```python
from build123d import *

# Parameters (mm, degrees)
F1_DEPTH = 6
F2_R     = 8
F2_R_2   = 7
F3_DEPTH = 5
F4_DEPTH = 26.3


with BuildPart() as f1:
    # F0 (on Front) → F1 (new body)
    with BuildSketch(Plane.XZ):
        Polygon((40, 0), (0, 0), (-40, 0), (-40, -29.434), (0, -29.434), (40, -29.434), align=None)
    extrude(amount=F1_DEPTH)

    # F2 (on face) → F3 (cut)
    with BuildSketch(Plane.XZ):
        with Locations((0, -8.284)):
            Circle(F2_R)
        with Locations((0, -8.284)):
            Circle(F2_R_2, mode=Mode.SUBTRACT)
    extrude(amount=F3_DEPTH, mode=Mode.SUBTRACT)

    # F2 (on face) → F4 (cut)
    with BuildSketch(Plane.XZ):
        with Locations((0, -8.284)):
            Circle(F2_R_2)
    extrude(amount=F4_DEPTH, mode=Mode.SUBTRACT)


solid = f1.part
```
Part model, mm, in its own coordinate system. A direction names the side the tool comes from. Coordinates: 2 decimals unless noted, no trailing zeros. Order: outer loops, then holes, each group sorted by start corner. A loop starts at its lowest first (then second) coordinate and runs counter-clockwise, first axis right, second up. Notation, with made-up numbers: (-25, 67.25) -> (8, 67.25) arc R26 cw to (8, 85.25) -> close; hole circle Ø2 at (68.25, 86.5). An arc over 180 degrees is marked (long way). Put each result on its own line as item: value. Start each with the question number.
(1) Probe line 1 along Z through (x, y) = (0, -2.15); line 2 along Z through (x, y) = (0, -5.4); line 3 along X through (y, z) = (-2.5, -9). List the from-to ranges inside material, lowest first. Write a range as [from, to].
(2) Mould opens along X. For faces 3 (the face through (40, -3, -15)), 4 (the face through (-1, 0, -18)), 5 (the face through (-1.7, -2.5, -16.1)) say: pulls with the +X half, pulls with the -X half, needs draft (parallel to the pull), parting line crosses it, or undercut.
(3) Band-saw the part on C-C (y = -1.3). Give the cut face in (x, z).
(4) Band-saw the part on B-B (x = 0). Give the cut face in (y, z), then the cut area to 3 significant figures.
(5) Which spindle directions (+Z, -Z, +X, -X, +Y, -Y) get a long thin tool onto all of the face, cutting with end or side? Do faces 1 (the face through (5, -5, -14)), 2 (the face through (-1, -3, -29.434)). Say none if no direction does.
(6) Band-saw the part on A-A (z = -14.5). Give the cut face in (x, y), then the cut area to 3 significant figures.
Determined:
1. line 1: z = [-29.43, -16.28], [-0.28, 0]
1. line 2: z = [-29.43, -15.28], [-1.28, 0]
1. line 3: x = [-40, -7.97], [7.97, 40]
2. face 3: pulls with the +X half
2. face 4: needs draft
2. face 5: undercut
3. outline: (-40, -29.43) -> (40, -29.43) -> (40, 0) -> (-40, 0) -> close; hole circle Ø16 at (0, -8.28)
4. outline: (-6, -29.43) -> (0, -29.43) -> (0, -16.28) -> (-5, -16.28) -> (-5, -15.28) -> (-6, -15.28) -> close; (-6, -1.28) -> (-5, -1.28) -> (-5, -0.28) -> (0, -0.28) -> (0, 0) -> (-6, 0) -> close
4. area: 82.6 mm²
5. face 1: +Y
5. face 2: -Z, +X, -X, +Y, -Y
6. outline: (-40, -6) -> (-3.22, -6) -> (-3.22, -5) -> (-5.04, -5) -> (-5.04, 0) -> (-40, 0) -> close; (3.22, -6) -> (40, -6) -> (40, 0) -> (5.04, 0) -> (5.04, -5) -> (3.22, -5) -> close
6. area: 423 mm²
